```python
from build123d import *

# Parameters (mm, degrees)
F1_R      = 7.5
F3_R      = 12.5
F3_R_2    = 7.5
F4_DEPTH  = 25
F5_DEPTH  = 25.0010001
F7_R      = 12.5
F8_DEPTH  = 12.5
F9_R      = 7.5
F10_DEPTH = 37.5010001


with BuildPart() as f2:
    # F2: sweep along a path in F0
    with BuildLine(Plane.XZ) as f2_path:
        Line((150, 0), (125, 0))
        ThreePointArc((125, 0), (77.8751511279, 2.6352872081), (31.3379403225, 10.5082872928))
        ThreePointArc((31.3379403225, 10.5082872928), (24.7317116593, 11.6259056014), (18.042064343, 12))
        Line((18.042064343, 12), (0, 12))
    # F1 (on Right) → F2 (sweep)
    with BuildSketch(Plane.YZ):
        with Locations((0, 12)):
            Circle(F1_R)
    sweep(path=f2_path.line)

    # F3 (on Top) → F4 (join)
    with BuildSketch(Plane.XY):
        Circle(F3_R)
        Circle(F3_R_2, mode=Mode.SUBTRACT)
        Circle(F3_R_2)
    extrude(amount=F4_DEPTH)

    # F3 (on Top) → F5 (cut, through all)
    with BuildSketch(Plane.XY):
        Circle(F3_R_2)
    extrude(amount=F5_DEPTH, mode=Mode.SUBTRACT)

    # F7 (on Top) → F8 (join, symmetric)
    with BuildSketch(Plane.XY):
        with Locations((150, 0)):
            Circle(F7_R)
    extrude(amount=F8_DEPTH, both=True)

    # F9 (on face) → F10 (cut, through all)
    with BuildSketch(Plane(origin=(0, 0, -12.5), x_dir=(1, 0, 0), z_dir=(0, 0, -1))):
        with Locations((150, 0)):
            Circle(F9_R)
    extrude(amount=-F10_DEPTH, mode=Mode.SUBTRACT)


solid = f2.part
```
Build history of the part. All positions in model axes, mm. A direction names the side the tool comes from. Give positions to 0.01 mm unless a question says otherwise; leave off trailing zeros. Order: outer loops, then holes, each group sorted by start corner. A loop starts at its lowest first (then second) coordinate and runs counter-clockwise, first axis right, second up. Notation, with made-up numbers: M -28.75,-22.75 L 27.25,-22.75 A32 cw 27.25,13.25 Z; hole C -3,26.5 d3. An arc over 180 degrees is marked long. Write item = value, one per line. Start each with the question number.
(1) Slice it at A-A on x = 150. Write the cut outline in (y, z), plus the area to 3 significant figures.
(2) Pin check, flat tips, straight feed: pin 1 Ø6 at (x, z) = (9, 1) entering from -Y; pin 2 Ø1 at (x, y) = (120.5, 6.5) entering from +Z; pin 3 Ø1 at (x, y) = (85.5, 6) entering from -Z. Stop position of each tip, or through.
(3) Which spindle directions (+Z, -Z, +X, -X, +Y, -Y) get a long thin tool onto all of the face, cutting with end or side? Do faces 1 (the cylindrical face through (132.395, 7.154, -2.253)), 2 (the flat face through (158, 0, 12.5)), 3 (the flat face through (0, -8, 0)), 4 (the flat face through (158, 0, -12.5)). Say none if no direction does.
(4) Slice it at B-B on y = 0. Write the cut outline in (x, z), plus the area to 3 significant figures.
(5) Probe L1, parallel to Y at x = 150, z = 3; L2, parallel to X at y = 3, z = 23; L3, parallel to Z at x = 3, y = 7. List the from-to ranges inside material, lowest first. Write a range as [from, to].
(6) Slice it at C-C on y = 9. Write the cut outline in (x, z).
(7) Two-plate mould, pull along Y, no slides. Class faces 5 (the cylindrical face through (156.93, 2.87, -0.18)), 6 (the flat face through (0, -8, 25)), 7 (the cylindrical face through (14.9, -5.5, 6.9)): released by +Y, released by -Y, zero draft, split by the parting line, or undercut.
Responses:
q1.outline = M -12.5,-12.5 L -7.5,-12.5 L -7.5,12.5 L -12.5,12.5 Z; M 7.5,-12.5 L 12.5,-12.5 L 12.5,12.5 L 7.5,12.5 Z
q1.area = 250 mm2
q2.pin_1 = -10.97
q2.pin_2 = 4.52
q2.pin_3 = -3.27
q3.face_1 = none
q3.face_2 = +Z, +X, +Y, -Y
q3.face_3 = -Z, -X, +Y, -Y
q3.face_4 = -Z, +X, -X, +Y, -Y
q4.outline = M -12.5,0 L -7.5,0 L -7.5,25 L -12.5,25 Z; M 7.5,0 L 12.5,0 L 12.5,4.5 L 18.04,4.5 A52.5 cw 29.68,3.19 A430.17 ccw 125,-7.5 L 137.5,-7.5 L 137.5,-12.5 L 142.5,-12.5 L 142.5,12.5 L 137.5,12.5 L 137.5,7.5 L 125,7.5 A415.17 cw 33,17.82 A67.5 ccw 18.04,19.5 L 12.5,19.5 L 12.5,25 L 7.5,25 Z; M 157.5,-12.5 L 162.5,-12.5 L 162.5,12.5 L 157.5,12.5 Z
q4.area = 2,390 mm2
q5.L1 = [-12.5, -7.5], [7.5, 12.5]
q5.L2 = [-12.13, -6.87], [6.87, 12.13]
q5.L3 = [0, 25]
q6.outline = M -8.67,0 L 8.67,0 L 8.67,25 L -8.67,25 Z; M 141.33,-12.5 L 158.67,-12.5 L 158.67,12.5 L 141.33,12.5 Z
q7.face_5 = undercut
q7.face_6 = zero draft
q7.face_7 = split by the parting line
